Read the model definition and answer for the solid it produces. Units are mm, in the model's axes. Coordinates: 2 decimals unless noted, no trailing zeros. Order: outer loops, then holes, each group sorted by start corner. A loop starts at its lowest first (then second) coordinate and runs counter-clockwise, first axis right, second up.
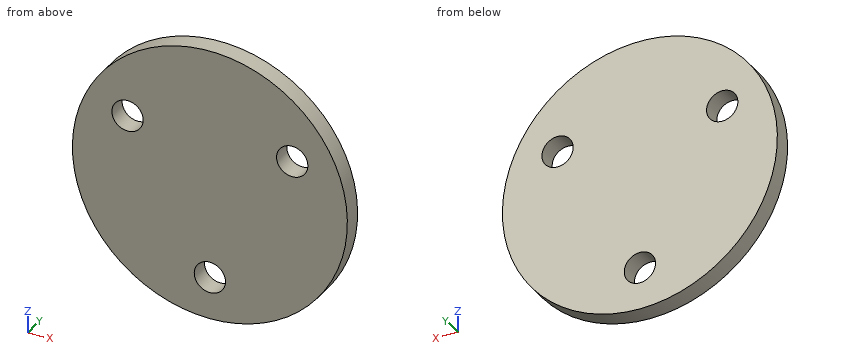
```python
from build123d import *

# Parameters (mm, degrees)
SKETCH1_R           = 11.938
BOSS_EXTRUDE1_DEPTH = 1.651
SKETCH2_R           = 1.3589
CUT_EXTRUDE1_DEPTH  = 1.651
CIRPATTERN1_COUNT   = 3


with BuildPart() as part:
    # Sketch1 → Boss-Extrude1 (new body)
    with BuildSketch(Plane(origin=(0, 0, 0), x_dir=(1, 0, 0), z_dir=(0, 1, 0))):
        with Locations(Location((0, 0, 0), (0, 0, 90))):
            Circle(SKETCH1_R)
    extrude(amount=BOSS_EXTRUDE1_DEPTH)

    # Sketch2 → Cut-Extrude1 (cut)
    with BuildSketch(Plane(origin=(0, 1.651, 0), x_dir=(1, 0, 0), z_dir=(0, 1, 0))):
        with Locations(Location((0, 8.255, 0), (0, 0, 270))):
            Circle(SKETCH2_R)
    cut_extrude1 = extrude(amount=-CUT_EXTRUDE1_DEPTH, mode=Mode.SUBTRACT)

    # CirPattern1: Cut-Extrude1 ×3 about axis
    cirpattern1_axis = Axis((0, 0, 0), (0, 1, 0))
    for i in range(1, CIRPATTERN1_COUNT):
        add(cut_extrude1.rotate(cirpattern1_axis, i * 360 / CIRPATTERN1_COUNT), mode=Mode.SUBTRACT)


solid = part.part
```
1) A flat-ended cylindrical pin translates along its axis: pin 1 Ø3 at (x, z) = (0, -8.255) entering from +Y. Find the tip coordinate at first contact, or state that the pin passes through.
A:
pin 1: stops at y = 1.65
2) A cutting plane is placed at A-A, the plane x = 0. Determine the outline of the cut face in (y, z), and give its area (3 significant figures).
A:
outline: (0, -11.94) - (1.65, -11.94) - (1.65, -9.61) - (0, -9.61) - close; (0, -6.9) - (1.65, -6.9) - (1.65, 11.94) - (0, 11.94) - close
area: 34.9 mm2
3) A cutting plane is placed at D-D, the plane z = -3.5. Determine the outline of the cut face in (x, y).
A:
outline: (-11.41, 0) - (11.41, 0) - (11.41, 1.65) - (-11.41, 1.65) - close
4) A cutting plane is placed at B-B, the plane y = 0.9. Determine the outline of the cut face in (x, z) (1 decimal), and give its area (3 significant figures).
A:
outline: circle Ø23.9 at (0, 0); hole circle Ø2.7 at (-7.1, 4.1); hole circle Ø2.7 at (0, -8.3); hole circle Ø2.7 at (7.1, 4.1)
area: 430 mm2
5) Straight lines are drawn through the part: line 1 (X direction, y = 1.45, z = 4.5); line 2 (X direction, y = 1, z = -8.75); line 3 (X direction, y = 0.3, z = 4.25). For each, find the intervals that lie inside material, in ascending order.
A:
line 1: x = -11.06 to -8.46, -5.84 to 5.84, 8.46 to 11.06
line 2: x = -8.12 to -1.27, 1.27 to 8.12
line 3: x = -11.16 to -8.5, -5.8 to 5.8, 8.5 to 11.16
6) A cutting plane is placed at C-C, the plane x = 5.25. Determine the outline of the cut face in (y, z).
A:
outline: (0, -10.72) - (1.65, -10.72) - (1.65, 10.72) - (0, 10.72) - close
